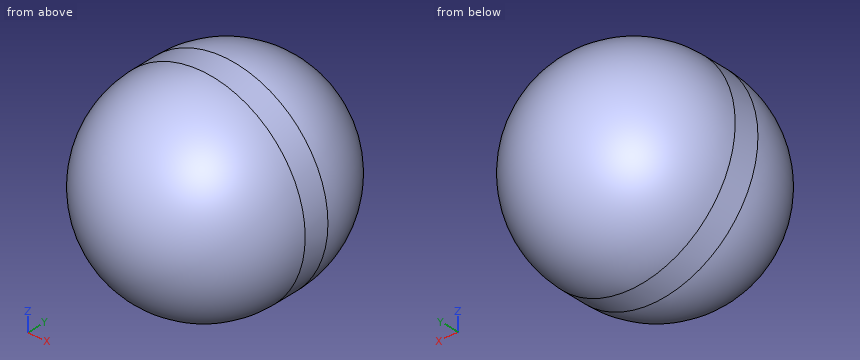
```python
from build123d import *

# Parameters (mm, degrees)
REVOLVE1_ANGLE      = 180
SKETCH2_R           = 30.897972145
BOSS_EXTRUDE1_DEPTH = 7.62
REVOLVE2_ANGLE      = 180


with BuildPart() as part:
    # Sketch1 → Revolve1 (revolve)
    with BuildSketch(Plane(origin=(0, 0, 0), x_dir=(1, 0, 0), z_dir=(0, 1, 0))):
        with BuildLine():
            Line((0, -30.897972145), (0, 30.897972145))
            ThreePointArc((0, 30.897972145), (30.897972145, 0), (0, -30.897972145))
        make_face()
    revolve(axis=Axis((0, 0, 30.897972145), (0, 0, -1)), revolution_arc=REVOLVE1_ANGLE)

    # Sketch2 → Boss-Extrude1 (add)
    with BuildSketch(Plane(origin=(0, 0, 0), x_dir=(1, 0, 0), z_dir=(0, 1, 0))):
        Circle(SKETCH2_R)
    extrude(amount=BOSS_EXTRUDE1_DEPTH)

    # Sketch3 → Revolve2 (revolve)
    with BuildSketch(Plane(origin=(0, 7.62, 0), x_dir=(1, 0, 0), z_dir=(0, 1, 0))):
        with BuildLine():
            Line((0, 30.897972145), (0, -30.897972145))
            ThreePointArc((0, -30.897972145), (30.897972145, 0), (0, 30.897972145))
        make_face()
    revolve(axis=Axis((0, 7.62, -30.897972145), (0, 0, 1)), revolution_arc=REVOLVE2_ANGLE)


solid = part.part
```
Verification items for the finished model (mm, model axes). Round coordinates to 2 decimals unless told otherwise and drop trailing zeros. Order: outer loops, then holes, each group sorted by start corner. A loop starts at its lowest first (then second) coordinate and runs counter-clockwise, first axis right, second up. Notation, with made-up numbers: (65.5, 52) - (84.5, 52) arc R27 ccw to (84.5, 90) - close; hole circle Ø3 at (-36, 40). An arc over 180 degrees is marked (long way). Use CSV: the item, a comma, the result in double quotes. Start each with the question number.
1) Section check B-B, the plane y = 1. Record the cut outline in (x, z).
2) Section check D-D, the plane y = -11. Record the cut outline in (x, z).
3) Section check C-C, the plane z = 21.5. Record the cut outline in (x, y), plus the area to 3 significant figures.
4) Thickness scan on L1, parallel to X at y = -7, z = -16; L2, parallel to X at y = 12, z = -9; L3, parallel to Z at x = 7, y = -0.5. Record the ranges inside material, lowest first.
5) Go/stop test with flat-tipped pins: P1, Ø3, axis at x = -14, z = -22.5, coming from the +Y side; P2, Ø1.5, axis at y = -8, z = -23, coming from the -X side; P3, Ø1, axis at y = -5.5, z = 16, coming from the -X side. Record where each tip stops, or that it passes through.
6) Section check A-A, the plane x = 0. Record the cut outline in (y, z), plus the area to 3 significant figures.
Answers:
1,outline,"circle Ø61.8 at (0, 0)"
2,outline,"circle Ø57.75 at (0, 0)"
3,outline,"(-22.19, 0) arc R22.19 ccw to (22.19, 0) - (22.19, 7.62) arc R22.19 ccw to (-22.19, 7.62) - close"
3,area,"1,890 mm²"
4,L1,"x = -25.49 to 25.49"
4,L2,"x = -29.23 to 29.23"
4,L3,"z = -30.09 to 30.09"
5,P1,"stops at y = 25.78"
5,P2,"stops at x = -19.94"
5,P3,"stops at x = -26.17"
6,outline,"(0, -30.9) - (7.62, -30.9) arc R30.9 ccw to (7.62, 30.9) - (0, 30.9) arc R30.9 ccw to start"
6,area,"3,470 mm²"
